Input: part model. Units: mm. Frame: model coordinates. A direction names the side the tool comes from. Round coordinates to 2 decimals unless told otherwise and drop trailing zeros. Loops run counter-clockwise (first coordinate to the right, second up) from the corner with the lowest first, then second, coordinate; pieces in that order, holes last.
(1) Cut plane C-C, the plane x = 143.5. Output: boundary loops of the cut face in (y, z).
(2) Access query for faces 4 (the face through (101.6, -44, 46)), 5 (the face through (107.95, -44, 51)), 6 (the face through (107.8, -88.9, 57.3)), 7 (the face through (-25, -44, 0)). Directions: +Z, -Z, +X, -X, +Y, -Y. A direction counts if a zero-diameter tool reaches every point of the face in a straight line with its end or side. Return the directions, or none.
(3) Line query: line 1 (X direction, y = -31.5, z = 31); line 2 (Z direction, x = 82, y = -67); line 3 (Z direction, x = 115.5, y = -64.5). Output: solid intervals per line, ascending.
(4) First-contact query: pin 1 Ø7 at (x, y) = (135.255, -17.145) entering from -Z; pin 2 Ø8 at (y, z) = (-63.5, 26) entering from +X; pin 3 Ø6 at (y, z) = (-58.5, 61) entering from -X; pin 4 Ø2 at (x, y) = (-18.5, -30) entering from +Z. Flat tips, straight axial feed; report the tip coordinate or a pass-through.
(5) Cut plane A-A, the plane z = 28.5. Output: boundary loops of the cut face in (x, y).
(6) Cut plane B-B, the plane y = -61. Output: boundary loops of the cut face in (x, z), and give its area (3 significant figures).
(7) Draft query along X for faces 1 (the face through (0, -44, 53)), 2 (the face through (53, -44, 97.79)), 3 (the face through (130, -44, -6.35)). Return one class per face: released by +X, released by -X, zero draft, split by the parting line, or undercut.
from build123d import *

# Parameters (mm, degrees)
F1_DEPTH = 88.9
F2_R     = 4.445
F3_DEPTH = 6.351


with BuildPart() as f1:
    # F0 (on Front) → F1 (new body)
    with BuildSketch(Plane.XZ):
        Polygon((0, 104.14), (0, 0), (-50.8, 0), (-50.8, -6.35), (6.35, -6.35), (6.35, 0), (6.35, 97.79), (101.6, 97.79), (101.6, 0), (101.6, -6.35), (158.75, -6.35), (158.75, 0), (107.95, 0), (107.95, 75.717971), (107.95, 104.14), align=None)
    extrude(amount=F1_DEPTH)

    # F2 (on face) → F3 (cut, through all)
    with BuildSketch(Plane.XY):
        with Locations((-27.305, -17.145)):
            Circle(F2_R)
        with Locations((-27.305, -71.755)):
            Circle(F2_R)
        with Locations((135.255, -71.755)):
            Circle(F2_R)
        with Locations((135.255, -17.145)):
            Circle(F2_R)
    extrude(amount=-F3_DEPTH, mode=Mode.SUBTRACT)


solid = f1.part
Reported:
1. outline: (-88.9, -6.35) - (0, -6.35) - (0, 0) - (-88.9, 0) - close
2. face 4: -Z, +Y, -Y
2. face 5: +Z, +X, +Y, -Y
2. face 6: +Z, -Z, +X, -X, -Y
2. face 7: +Z, -X, +Y, -Y
3. line 1: x = 0 to 6.35, 101.6 to 107.95
3. line 2: z = 97.79 to 104.14
3. line 3: z = -6.35 to 0
4. pin 1: passes through
4. pin 2: stops at x = 107.95
4. pin 3: stops at x = 0
4. pin 4: stops at z = 0
5. outline: (0, -88.9) - (6.35, -88.9) - (6.35, 0) - (0, 0) - close; (101.6, -88.9) - (107.95, -88.9) - (107.95, 0) - (101.6, 0) - close
6. outline: (-50.8, -6.35) - (6.35, -6.35) - (6.35, 97.79) - (101.6, 97.79) - (101.6, -6.35) - (158.75, -6.35) - (158.75, 0) - (107.95, 0) - (107.95, 104.14) - (0, 104.14) - (0, 0) - (-50.8, 0) - close
6. area: 2,650 mm2
7. face 1: released by -X
7. face 2: undercut
7. face 3: zero draft
